Drawing for the job (mm, zero at the part's lowest x, y, z). A direction names the side the tool comes from. Coordinates: 2 decimals unless noted, no trailing zeros. Write each loop counter-clockwise with the first axis right and the second up, starting at its lowest first coordinate (ties: lowest second). Pieces come first, ordered by that corner, then holes. Notation, with made-up numbers: (1, 57) -> (54, 57) arc R27 ccw to (54, 93) -> close; hole circle Ø9 at (-30, 26). An arc over 180 degrees is marked (long way). Answer as CSV lines item,"result".
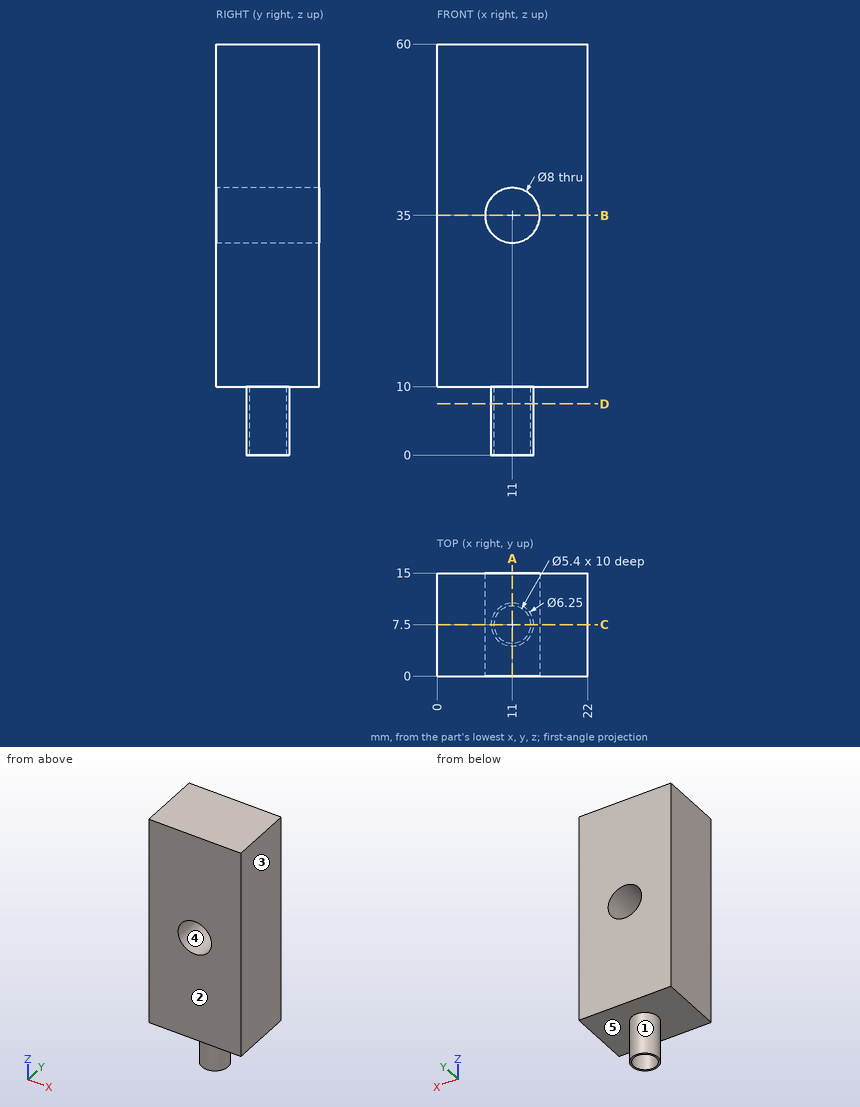
Item 1: Saw through at D-D on z = 7.5. Give the cut face in (x, y) (3 decimals), and give its area (3 significant figures).
Answer below:
outline,"circle Ø6.25 at (11, 7.5); hole circle Ø5.4 at (11, 7.5)"
area,"7.78 mm2"
Item 2: Saw through at C-C on y = 7.5. Give the cut face in (x, z) (3 decimals), and give its area (3 significant figures).
Answer below:
outline,"(0, 10) -> (7.875, 10) -> (7.875, 0) -> (8.3, 0) -> (8.3, 10) -> (13.7, 10) -> (13.7, 0) -> (14.125, 0) -> (14.125, 10) -> (22, 10) -> (22, 60) -> (0, 60) -> close; hole circle Ø8 at (11, 35)"
area,"1,060 mm2"
Item 3: Saw through at A-A on x = 11. Give the cut face in (y, z) (3 decimals).
Answer below:
outline,"(0, 10) -> (4.375, 10) -> (4.375, 0) -> (4.8, 0) -> (4.8, 10) -> (10.2, 10) -> (10.2, 0) -> (10.625, 0) -> (10.625, 10) -> (15, 10) -> (15, 31) -> (0, 31) -> close; (0, 39) -> (15, 39) -> (15, 60) -> (0, 60) -> close"
Item 4: Saw through at B-B on z = 35. Give the cut face in (x, y), and give its area (3 significant figures).
Answer below:
outline,"(0, 0) -> (7, 0) -> (7, 15) -> (0, 15) -> close; (15, 0) -> (22, 0) -> (22, 15) -> (15, 15) -> close"
area,"210 mm2"
Item 5: Two-plate mould, pull along Z, no slides. Class the marked faces 3, 4 and 5: pulls with the +Z half, pulls with the -Z half, needs draft (parallel to the pull), parting line crosses it, or undercut.
Answer below:
face 3,"needs draft"
face 4,"undercut"
face 5,"pulls with the -Z half"
Item 6: 3-axis set-ups, long thin cutter, end or side, ignore diameter. For the marked faces 1 and 2: which of +Z, -Z, +X, -X, +Y, -Y reach the whole face in a straight line?
Answer below:
face 1,"-Z"
face 2,"+Z, -Z, +X, -X, -Y"
Item 7: Wall check: line 1 (Y direction, x = 11, z = 5.75) (3 decimals); line 2 (X direction, y = 10, z = 35); line 3 (Z direction, x = 3.5, y = 4.5). Give the ranges that are in metal, low to high. Write a range as from..to.
Answer below:
line 1,"y = 4.375..4.8, 10.2..10.625"
line 2,"x = 0..7, 15..22"
line 3,"z = 10..60"
